Here's the drawing with two shaded views (mm, measured from the low corner). I have some questions. Coordinates: 2 decimals unless noted, no trailing zeros. Loops run counter-clockwise (first coordinate to the right, second up) from the corner with the lowest first, then second, coordinate; pieces in that order, holes last.
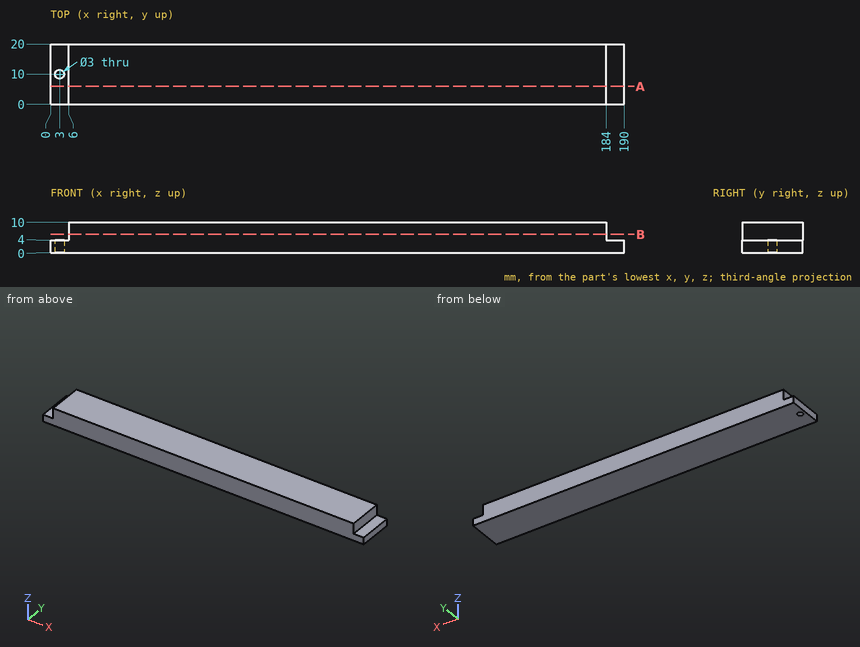
(1) I'm going to push flat-ended pins straight in: pin 1 (1.8 mm diameter, centred on x = 188.5, y = 8.5, fed in from +Z); pin 2 (3 mm diameter, centred on y = 9, z = 6.5, fed in from +X); pin 3 (3 mm diameter, centred on y = 5.5, z = 8, fed in from -X). Where does each tip first touch, or does it pass through?
Check values:
pin 1: stops at z = 4
pin 2: stops at x = 184
pin 3: stops at x = 6
(2) I want a section at A-A on y = 6. Write out the boundary of the cut face in (x, z).
Check values:
outline: (0, 0) - (190, 0) - (190, 4) - (184, 4) - (184, 10) - (6, 10) - (6, 4) - (0, 4) - close
(3) If I drill on probe 1 along Y at (x, z) = (3, 1.15); probe 2 along X at (y, z) = (10.25, 1.5); probe 3 along X at (y, z) = (12.25, 7.25), over which ranges is the centre line in solid material (lowest first)?
Check values:
probe 1: y = 0 to 8.5, 11.5 to 20
probe 2: x = 0 to 1.52, 4.48 to 190
probe 3: x = 6 to 184
(4) I want a section at B-B on z = 6. Write out the boundary of the cut face in (x, y), then the cut area to 3 significant figures.
Check values:
outline: (6, 0) - (184, 0) - (184, 20) - (6, 20) - close
area: 3,560 mm2
